Verification items for the finished model (mm, model axes). Give positions to 0.01 mm unless a question says otherwise; leave off trailing zeros. Order: outer loops, then holes, each group sorted by start corner. A loop starts at its lowest first (then second) coordinate and runs counter-clockwise, first axis right, second up.
from build123d import *

# Parameters (mm, degrees)
SALIENTE_EXTRUIR1_DEPTH = 2.44


with BuildPart() as part:
    # Croquis1 → Saliente-Extruir1 (new body)
    with BuildSketch(Plane(origin=(0, 0, 0), x_dir=(0, 0, -1), z_dir=(1, 0, 0))):
        with BuildLine():
            Line((26, -55.56), (26, -55.153543901))
            ThreePointArc((26, -55.153543901), (0, 31), (-26, -55.153543901))
            Line((-26, -55.153543901), (-26, -55.56))
            Line((-26, -55.56), (-35, -55.56))
            Line((-35, -55.56), (-35, -58))
            Line((-35, -58), (-45, -58))
            Line((-45, -58), (-45, -55.56))
            Line((-45, -55.56), (-59, -55.56))
            Line((-59, -55.56), (-59, 55.56))
            Line((-59, 55.56), (-35, 55.56))
            Line((-35, 55.56), (-35, 58))
            Line((-35, 58), (-15, 58))
            Line((-15, 58), (-15, 55.56))
            Line((-15, 55.56), (15, 55.56))
            Line((15, 55.56), (15, 58))
            Line((15, 58), (35, 58))
            Line((35, 58), (35, 55.56))
            Line((35, 55.56), (59, 55.56))
            Line((59, 55.56), (59, -55.56))
            Line((59, -55.56), (45, -55.56))
            Line((45, -55.56), (45, -58))
            Line((45, -58), (35, -58))
            Line((35, -58), (35, -55.56))
            Line((35, -55.56), (26, -55.56))
        make_face()
    extrude(amount=SALIENTE_EXTRUIR1_DEPTH)


solid = part.part
(1) Release check for a two-part mould opening along Z. For faces 1 (the cylindrical face through (1.2, 30.97, -1.68)), 2 (the flat face through (2.44, 39, -1)) record: pulls with the +Z half, pulls with the -Z half, needs draft (parallel to the pull), parting line crosses it, or undercut.
Solved:
face 1: undercut
face 2: needs draft
(2) Section check C-C, the plane x = 0.4. Enter the section's corners in (y, z).
Solved:
outline: (-58, -45) - (-55.56, -45) - (-55.56, -59) - (55.56, -59) - (55.56, -35) - (58, -35) - (58, -15) - (55.56, -15) - (55.56, 15) - (58, 15) - (58, 35) - (55.56, 35) - (55.56, 59) - (-55.56, 59) - (-55.56, 45) - (-58, 45) - (-58, 35) - (-55.56, 35) - (-55.56, 26) - (-55.15, 26) arc R47 cw (long way) to (-55.15, -26) - (-55.56, -26) - (-55.56, -35) - (-58, -35) - close
(3) Go/stop test with flat-tipped pins: pin 1 (1.2 mm diameter, centred on x = 1, z = 51, fed in from -Y); pin 2 (1.2 mm diameter, centred on x = 1.5, y = 56.5, fed in from -Z); pin 3 (1 mm diameter, centred on y = 29.5, z = -10.5, fed in from -X); pin 4 (1.2 mm diameter, centred on x = 1, z = -43.5, fed in from +Y). Record where each tip stops, or that it passes through.
Solved:
pin 1: stops at y = -55.56
pin 2: stops at z = -35
pin 3: stops at x = 0
pin 4: stops at y = 55.56
(4) Scan lines: line 1 (Y direction, x = 1.3, z = 0); line 2 (Z direction, x = 0.95, y = -16); line 3 (Z direction, x = 1.7, y = -25.5). Record each from-to range of solid material in increasing order.
Solved:
line 1: y = 31 to 55.56
line 2: z = -59 to -47, 47 to 59
line 3: z = -59 to -46.03, 46.03 to 59
(5) Section check A-A, the plane y = -16. Enter the section's corners in (x, z).
Solved:
outline: (0, -59) - (2.44, -59) - (2.44, -47) - (0, -47) - close; (0, 47) - (2.44, 47) - (2.44, 59) - (0, 59) - close
(6) Section check B-B, the plane z = -28.5. Enter the section's corners in (x, y), then the cut area to 3 significant figures.
Solved:
outline: (0, -55.56) - (2.44, -55.56) - (2.44, -53.37) - (0, -53.37) - close; (0, 21.37) - (2.44, 21.37) - (2.44, 58) - (0, 58) - close
area: 94.7 mm2
(7) Section check D-D, the plane z = 0. Enter the section's corners in (x, y), then the cut area to 3 significant figures.
Solved:
outline: (0, 31) - (2.44, 31) - (2.44, 55.56) - (0, 55.56) - close
area: 59.9 mm2
